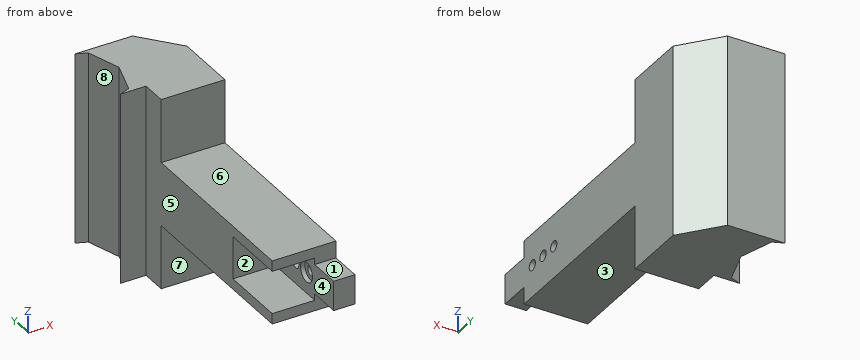
Autodesk Inventor part; units mm, degrees
ref_plane "Work Plane1" through (0, 0, -15) normal (0, 0, 1) x (1, 0, 0)
ref_plane "YZ Plane" through (0, 0, 0) normal (1, 0, 0) x (0, 1, 0)
ref_plane "XZ Plane" through (0, 0, 0) normal (0, 1, 0) x (-1, 0, 0)
sketch "Sketch1" plane through (0, 0, 0) normal (0, 0, 1) x (1, 0, 0)
  line L0 (0, 0) -> (25, 0)
  line L1 (25, 0) -> (25, 40)
  line L2 (25, 40) -> (0, 40)
  line L3 (0, 40) -> (0, 0)
  dimension "d1" = 25
  dimension "d2" = 40
  dimension "d3" = 25
extrude "Extrusion1" add sketch "Sketch1" against normal blind 30
sketch "Sketch2" plane through (25, 0, 0) normal (1, 0, 0) x (0, 0, -1)
  line L0 (0, 0) -> (30, 0)
  circle A0 centre (15, 6.56) radius 2.46
extrude "Extrusion2" cut sketch "Sketch2" against normal blind 30
sketch "Sketch3" plane through (0, 0, 0) normal (-1, 0, 0) x (0, 0, 1)
  line L0 (0, 0) -> (-30, 0)
  line L1 (-25.05, 0) -> (-4.95, 0)
  line L2 (-4.95, 0) -> (-4.95, 33.12)
  line L3 (-4.95, 33.12) -> (-25.05, 33.12)
  line L4 (-25.05, 33.12) -> (-25.05, 0)
  dimension "d11" = 20.1
extrude "Extrusion3" cut sketch "Sketch3" against normal blind 20
sketch "Sketch4" plane through (0, 0, 0) normal (0, -1, 0) x (1, 0, 0)
  line L0 (20, -4.95) -> (20, -25.05)
  line L1 (20, -15) -> (25, -15)
  line L2 (25, 0) -> (25, -30)
  line L3 (20, -8.025) -> (25, -8.025)
  line L4 (25, -8.025) -> (25, -21.975)
  line L5 (25, -21.975) -> (20, -21.975)
  line L6 (20, -21.975) -> (20, -8.025)
  line L7 (20, -8.025) -> (25, -21.975) construction
  line L8 (25, -8.025) -> (20, -21.975) construction
  line L9 (25, -12.54) -> (25, -17.46)
  point P0 (0, 0)
  point P1 (22.5, -15)
  dimension "d14" = 13.95
extrude "Extrusion4" add sketch "Sketch4" along normal blind 15
sketch "Sketch5" plane through (20, 0, 0) normal (-1, 0, 0) x (0, 0, 1)
  circle A0 centre (-15, 6.56) radius 2.46
  circle A1 centre (-15, 6.56) radius 4.7025
  circle A2 centre (-15, 6.56) radius 2.46
  circle A3 centre (-15, 6.56) radius 2.46
  point P0 (0, 0)
  dimension "d17" = 9.405
extrude "Extrusion5" cut sketch "Sketch5" against normal blind 2.1
sketch "Sketch6" plane through (25, 0, 0) normal (1, 0, 0) x (0, 0, -1)
  circle A0 centre (15, 6.56) radius 4.7025
  line L0 (15, 6.56) -> (15, 23.56)
  circle A1 centre (15, 23.56) radius 2.46
  point P0 (0, 0)
  dimension "d20" = 17
  dimension "d21" = 4.92
extrude "Extrusion6" cut sketch "Sketch6" against normal blind 10 contours A1
sketch "Sketch7" plane through (20, 0, 0) normal (-1, 0, 0) x (0, 0, 1)
  circle A0 centre (-15, 23.56) radius 2.46
  circle A1 centre (-15, 23.56) radius 4.7025
  point P0 (0, 0)
  dimension "d24" = 9.405
extrude "Extrusion7" cut sketch "Sketch7" against normal blind 2.1
sketch "Sketch9" plane through (25, 0, 0) normal (1, 0, 0) x (0, 0, -1)
  circle A0 centre (15, 6.56) radius 2.46
  circle A1 centre (15, 6.56) radius 2.46
  circle A2 centre (15, 23.56) radius 2.46
  circle A3 centre (15, 23.56) radius 2.46
  line L0 (30, 40) -> (30, 0)
  line L1 (30, 0) -> (30, 40)
  line L2 (30, 40) -> (0, 40)
  line L3 (0, 40) -> (0, 0)
  line L4 (0, 0) -> (8.025, 0)
  line L5 (21.975, 0) -> (21.975, -15)
  line L6 (21.975, -15) -> (8.025, -15)
  line L7 (8.025, -15) -> (8.025, 0)
  line L8 (0, 0) -> (8.025, 0)
  line L9 (21.975, 0) -> (30, 0)
extrude "Extrusion8" add sketch "Sketch9" along normal blind 5
sketch "Sketch10" plane through (0, 40, 0) normal (0, 1, 0) x (1, 0, 0)
  line L0 (0, 30) -> (30, 30)
  line L1 (30, 0) -> (0, 0)
  line L2 (0, 30) -> (30, 30)
  line L3 (30, 30) -> (30, 0)
  line L4 (30, 0) -> (0, 0)
  line L5 (0, 0) -> (0, 30)
extrude "Extrusion9" add sketch "Sketch10" along normal blind 30
sketch "Sketch12" plane through (30, 0, 0) normal (1, 0, 0) x (0, 0, -1)
  circle A0 centre (15, 6.56) radius 2.46
  line L0 (15, 6.56) -> (15, 15.06)
  circle A1 centre (15, 15.06) radius 2.525
  point P0 (0, 0)
  dimension "d31" = 8.5
  dimension "d33" = 5.05
extrude "Extrusion10" cut sketch "Sketch12" against normal blind 30 contours A1
sketch "Sketch14" plane through (0, 0, 0) normal (0, 0, 1) x (1, 0, 0)
  line L0 (30, 70) -> (0, 70)
  line L1 (0, 70) -> (0, 85)
  line L2 (30, 0) -> (30, 70)
  line L3 (30, 118) -> (30, 70)
  line L4 (30, 105) -> (30, 100)
  line L5 (-7, 134) -> (-12, 136)
  line L6 (-7, 102) -> (-12, 100)
  line L7 (-7, 102) -> (-2, 118)
  line L8 (-2, 118) -> (-7, 134)
  line L9 (15, 136) -> (30, 118)
  line L10 (-12, 136) -> (15, 136)
  line L11 (0, 85) -> (0, 100)
  line L12 (0, 100) -> (-12, 100)
  point P0 (0, 0)
  dimension "d82" = 12
extrude "Extrusion12" add sketch "Sketch14" against normal blind 30
sketch "Sketch15" plane through (0, 0, -25.05) normal (-1, 0, 0) x (0, 0, 1)
  line L0 (0, 33.12) -> (20.1, 33.12)
  line L1 (20.1, 33.12) -> (20.1, 0)
  line L2 (0, 33.12) -> (20.1, 33.12)
  line L3 (20.1, 33.12) -> (20.1, 31.1)
  line L4 (20.1, 31.1) -> (0, 31.1)
  line L5 (0, 31.1) -> (0, 33.12)
  point P0 (25.05, 0)
  dimension "d57" = 2.02
extrude "Extrusion13" add sketch "Sketch15" against normal blind 20
sketch "Sketch23" plane through (0, 0, 0) normal (0, 0, 1) x (1, 0, 0)
  line L0 (0, 100) -> (-12, 100)
  line L1 (0, 100) -> (-12, 100)
  line L2 (-12, 100) -> (-7, 102)
  line L3 (-12, 100) -> (-7, 102)
  line L4 (-7, 102) -> (-2, 118)
  line L5 (-7, 102) -> (-2, 118)
  line L6 (-2, 118) -> (-7, 134)
  line L7 (-2, 118) -> (-7, 134)
  line L8 (-12, 136) -> (15, 136)
  line L9 (-7, 134) -> (-12, 136)
  line L10 (-12, 136) -> (15, 136)
  line L11 (15, 136) -> (30, 118)
  line L12 (15, 136) -> (30, 118)
  line L13 (30, 118) -> (30, 88)
  line L14 (30, 0) -> (30, 118)
  line L15 (30, 88) -> (0, 88)
  line L16 (0, 88) -> (0, 100)
  point P0 (0, 0)
  dimension "d83" = 30
  dimension "d84" = 30
extrude "Extrusion14" add sketch "Sketch23" along normal blind 30
ref_plane "Work Plane1" through (0, 0, -15) normal (0, 0, 1) x (1, 0, 0)
mirror "Mirror1" about plane through (0, 0, -15) normal (0, 0, 1) of "Extrusion14"
properties part number "rec_b_32mm_x_90mm"
Can you work these out from the model? Positions are in its coordinate system, mm. Face numbers are marked on the shaded views. A direction names the side the tool comes from. Coordinates: 2 decimals unless noted, no trailing zeros. Write each loop counter-clockwise with the first axis right and the second up, starting at its lowest first coordinate (ties: lowest second). Pieces come first, ordered by that corner, then holes.
Q1. For P1, Ø13, axis at x = -7.5, z = -28, coming from the -Y side; P2, Ø24, axis at x = 20, z = 15.5, coming from the -Y side; P3, Ø3, axis at x = 23.5, y = -10, coming from the +Z side (3 decimals), each with a flat end and sliding along its axis, tell me the tip position at first contact or that it passes through.
Results found:
P1: stops at y = 100
P2: stops at y = 88
P3: stops at z = -8.025
Q2. Which directions (+Z, -Z, +X, -X, +Y, -Y) give clear straight access to the entire face, cutting with the end or side of a thin tool? Please do the marked faces 4, 5, 6, 7 and 8.
Results found:
face 4: -X, -Y
face 5: +Z, -Z, -X, -Y
face 6: +Z, +X, -X, -Y
face 7: -Z, +X, -X, -Y
face 8: +Z, -Z, -X
Q3. Imagine slicing it at C-C, the plane z = -15. Count the separate pieces of the cut face and the enclosed holes in it, plus the area to 3 significant figures.
Results found:
separate pieces: 4
enclosed holes: 0
area: 3,490 mm2
Q4. Imagine slicing it at B-B, the plane y = 15.06. List the corners of the cut face in (x, z) for me (3 decimals).
Results found:
outline: (0, -30) - (30, -30) - (30, -17.525) - (20, -17.525) - (20, -25.05) - (0, -25.05) - close; (0, -4.95) - (20, -4.95) - (20, -12.475) - (30, -12.475) - (30, 0) - (0, 0) - close
Q5. If we mould it in two halves opening along Z, with no side actions, what happens to the marked faces 1, 2 and 3? For each: +Z half, -Z half, draft (parallel to the pull), parting line (faces both ways), or undercut.
Results found:
face 1: +Z half
face 2: undercut
face 3: -Z half
Q6. Imagine slicing it at A-A, the plane x = -3.5. List the corners of the cut face in (y, z) for me, plus the area to 3 significant figures.
Results found:
outline: (100, -60) - (113.2, -60) - (113.2, 30) - (100, 30) - close; (122.8, -60) - (136, -60) - (136, 30) - (122.8, 30) - close
area: 2,380 mm2
Q7. Imagine slicing it at D-D, the plane x = 17.5. List the corners of the cut face in (y, z) for me, plus the area to 3 significant figures.
Results found:
outline: (0, -30) - (88, -30) - (88, -60) - (133, -60) - (133, 30) - (88, 30) - (88, 0) - (0, 0) - (0, -4.95) - (31.1, -4.95) - (31.1, -25.05) - (0, -25.05) - close
area: 6,060 mm2
Q8. Please list where these lines run through material, in increasing order: L1, parallel to Y at x = 26.5, z = -15 (3 decimals); L2, parallel to Z at x = 21, y = 6; L3, parallel to Z at x = 28, y = 23.56.
Results found:
L1: y = -15 to 4.1, 9.02 to 12.535, 17.585 to 21.1, 26.02 to 122.2
L2: z = -30 to -19.67, -10.33 to 0
L3: z = -30 to -17.46, -12.54 to 0
